Read the model definition and answer for the solid it produces. Units are mm, in the model's axes. A direction names the side the tool comes from. Give positions to 0.01 mm unless a question says otherwise; leave off trailing zeros. Loops run counter-clockwise (first coordinate to the right, second up) from the corner with the lowest first, then second, coordinate; pieces in that order, holes last. Notation, with made-up numbers: (-23, 84) -> (29, 84) arc R31 ccw to (29, 113) -> close; hole circle Ø4 at (-19, 30.25). An arc over 180 degrees is marked (long way). Write each question's results on one line, items separated by ' | '. Start each with the question number.
Item 1: Find the intervals of material crossed by line 1 (X direction, y = 16, z = 0); line 2 (X direction, y = 1.5, z = 8.5); line 3 (Z direction, x = 9.25, y = 11.5), in increasing order.
Item 2: Determine the mould class of faces 3 (the flat face through (10, 11, 10)), 4 (the flat face through (7.465, -13.681, 4.332)) for opening direction Y: +Y half, -Y half, draft (parallel to the pull), parting line (faces both ways), or undercut.
Item 3: Each of these flat-tipped pins is pushed along its axis until it touches: P1, Ø1, axis at x = 3.5, z = 3.5, coming from the -Y side; P2, Ø5, axis at x = 5, y = -15, coming from the +Z side; P3, Ø5, axis at x = 2.5, y = 13, coming from the +Z side. Where does it stop, or does it pass through?
Item 4: Section D-D on x = 2.5 is taken. Write down the section's boundary in (y, z), and give its area (3 significant figures).
Item 5: Section A-A on z = 0 is taken. Write down the section's boundary in (x, y).
Item 6: Section B-B on y = 0 is taken. Write down the section's boundary in (x, z).
Item 7: Section C-C on x = 6.75 is taken. Write down the section's boundary in (y, z).
Item 8: Which of the six approach directions +Z, -Z, +X, -X, +Y, -Y give full straight-line access (tool end or side, diameter ignored) to faces 1 (the cylindrical face through (1.9, 11.1, 0)), 2 (the flat face through (7.465, 13.54, -4.348))?
```python
from build123d import *

# Parameters (mm, degrees)
SKETCH2_R           = 19.05
BOSS_EXTRUDE1_DEPTH = 5
BOSS_EXTRUDE2_DEPTH = 5
SKETCH6_R           = 3.05
CUT_EXTRUDE1_DEPTH  = 25
SKETCH8_R           = 0.6
CUT_EXTRUDE4_DEPTH  = 25


with BuildPart() as part:
    # Sketch2 → Boss-Extrude1 (new body)
    with BuildSketch(Plane(origin=(0, 0, 0), x_dir=(0, 0, -1), z_dir=(1, 0, 0))):
        Circle(SKETCH2_R)
    extrude(amount=BOSS_EXTRUDE1_DEPTH)

    # Sketch4 → Boss-Extrude2 (add)
    with BuildSketch(Plane(origin=(5, 0, 0), x_dir=(0, 0, -1), z_dir=(1, 0, 0))):
        with BuildLine():
            Line((4.886596437, 8.552407571), (3.793697076, 18.668432245))
            ThreePointArc((3.793697076, 18.668432245), (13.529522994, 13.410984586), (18.701093352, 3.629270922))
            Line((18.701093352, 3.629270922), (8.502967267, 4.972127076))
            ThreePointArc((8.502967267, 4.972127076), (6.929986014, 6.999842416), (4.886596437, 8.552407571))
        make_face()
        with BuildLine():
            Line((-4.886596437, 8.552407571), (-3.793697076, 18.668432245))
            ThreePointArc((-3.793697076, 18.668432245), (-13.529522994, 13.410984586), (-18.701093352, 3.629270922))
            Line((-18.701093352, 3.629270922), (-8.502967267, 4.972127076))
            ThreePointArc((-8.502967267, 4.972127076), (-6.929986014, 6.999842416), (-4.886596437, 8.552407571))
        make_face()
        with BuildLine():
            Line((-8.502967267, -4.972127076), (-18.701093352, -3.629270922))
            ThreePointArc((-18.701093352, -3.629270922), (-13.529522994, -13.410984586), (-3.793697076, -18.668432245))
            Line((-3.793697076, -18.668432245), (-4.886596437, -8.552407571))
            ThreePointArc((-4.886596437, -8.552407571), (-6.929986014, -6.999842416), (-8.502967267, -4.972127076))
        make_face()
        with BuildLine():
            Line((4.886596437, -8.552407571), (3.793697076, -18.668432245))
            ThreePointArc((3.793697076, -18.668432245), (13.529522994, -13.410984586), (18.701093352, -3.629270922))
            Line((18.701093352, -3.629270922), (8.502967267, -4.972127076))
            ThreePointArc((8.502967267, -4.972127076), (6.929986014, -6.999842416), (4.886596437, -8.552407571))
        make_face()
    extrude(amount=BOSS_EXTRUDE2_DEPTH)

    # Sketch6 → Cut-Extrude1 (cut)
    with BuildSketch(Plane.ZY):
        Circle(SKETCH6_R)
    extrude(amount=-CUT_EXTRUDE1_DEPTH, mode=Mode.SUBTRACT)

    # Sketch8 → Cut-Extrude4 (cut, symmetric)
    with BuildSketch(Plane(origin=(0, 0, 0), x_dir=(1, 0, 0), z_dir=(0, 1, 0))):
        with Locations((2.5, 0)):
            Circle(SKETCH8_R)
    extrude(amount=CUT_EXTRUDE4_DEPTH, both=True, mode=Mode.SUBTRACT)


solid = part.part
```
Findings:
1) line 1: 0 to 1.9, 3.1 to 5 | line 2: 0 to 5 | line 3: -15.19 to -4.57, 4.57 to 15.19
2) face 3: draft | face 4: undercut
3) P1: y = -18.81 | P2: z = 14.38 | P3: z = 15.9
4) outline: (-19.04, -0.6) arc R19.05 ccw to (19.04, -0.6) -> (2.99, -0.6) arc R3.05 cw to (-2.99, -0.6) -> close; (-19.04, 0.6) -> (-2.99, 0.6) arc R3.05 cw to (2.99, 0.6) -> (19.04, 0.6) arc R19.05 ccw to start | area: 1,070 mm2
5) outline: (0, -19.05) -> (1.9, -19.05) -> (1.9, -3.05) -> (0, -3.05) -> close; (0, 3.05) -> (1.9, 3.05) -> (1.9, 19.05) -> (0, 19.05) -> close; (3.1, -19.05) -> (5, -19.05) -> (5, -3.05) -> (3.1, -3.05) -> close; (3.1, 3.05) -> (5, 3.05) -> (5, 19.05) -> (3.1, 19.05) -> close
6) outline: (0, -19.05) -> (5, -19.05) -> (5, -3.05) -> (0, -3.05) -> close; (0, 3.05) -> (5, 3.05) -> (5, 19.05) -> (0, 19.05) -> close
7) outline: (-18.67, -3.79) arc R19.05 ccw to (-3.63, -18.7) -> (-4.97, -8.5) arc R9.85 cw to (-8.55, -4.89) -> close; (-18.67, 3.79) -> (-8.55, 4.89) arc R9.85 cw to (-4.97, 8.5) -> (-3.63, 18.7) arc R19.05 ccw to start; (3.63, -18.7) arc R19.05 ccw to (18.67, -3.79) -> (8.55, -4.89) arc R9.85 cw to (4.97, -8.5) -> close; (3.63, 18.7) -> (4.97, 8.5) arc R9.85 cw to (8.55, 4.89) -> (18.67, 3.79) arc R19.05 ccw to start
8) face 1: +Y, -Y | face 2: +X
